from build123d import *

# Parameters (mm, degrees)
SKETCH1_W           = 15
SKETCH1_H           = 5
BOSS_EXTRUDE1_DEPTH = 9.75
SKETCH2_R           = 1.5
CUT_EXTRUDE1_DEPTH  = 4
SKETCH3_W           = 5
SKETCH3_H           = 0.5
BOSS_EXTRUDE2_DEPTH = 4
SKETCH4_W           = 5
SKETCH4_H           = 0.5
BOSS_EXTRUDE3_DEPTH = 4
SKETCH5_R           = 1
CUT_EXTRUDE2_DEPTH  = 4


with BuildPart() as part:
    # Sketch1 → Boss-Extrude1 (new body)
    with BuildSketch(Plane(origin=(0, 0, 0), x_dir=(1, 0, 0), z_dir=(0, 1, 0))):
        with Locations((-0.341726619, 0)):
            Rectangle(SKETCH1_W, SKETCH1_H)
    extrude(amount=BOSS_EXTRUDE1_DEPTH)

    # Sketch2 → Cut-Extrude1 (cut)
    with BuildSketch(Plane(origin=(0, 9.75, 0), x_dir=(1, 0, 0), z_dir=(0, 1, 0))):
        with Locations((-4.091726619, 0)):
            Circle(SKETCH2_R)
        with Locations((3.408273381, 0)):
            Circle(SKETCH2_R)
    extrude(amount=-CUT_EXTRUDE1_DEPTH, mode=Mode.SUBTRACT)

    # Sketch3 → Boss-Extrude2 (add)
    with BuildSketch(Plane(origin=(7.158273381, 0, 0), x_dir=(0, 0, -1), z_dir=(1, 0, 0))):
        with Locations((0, 0.25)):
            Rectangle(SKETCH3_W, SKETCH3_H)
    extrude(amount=BOSS_EXTRUDE2_DEPTH)

    # Sketch4 → Boss-Extrude3 (add)
    with BuildSketch(Plane.ZY.offset(7.841726619)):
        with Locations((0, 0.25)):
            Rectangle(SKETCH4_W, SKETCH4_H)
    extrude(amount=BOSS_EXTRUDE3_DEPTH)

    # Sketch5 → Cut-Extrude2 (cut)
    with BuildSketch(Plane(origin=(0, 0.5, 0), x_dir=(1, 0, 0), z_dir=(0, 1, 0))):
        with Locations((-9.841726619, 0)):
            Circle(SKETCH5_R)
        with Locations((9.158273381, 0)):
            Circle(SKETCH5_R)
    extrude(amount=-CUT_EXTRUDE2_DEPTH, mode=Mode.SUBTRACT)


solid = part.part
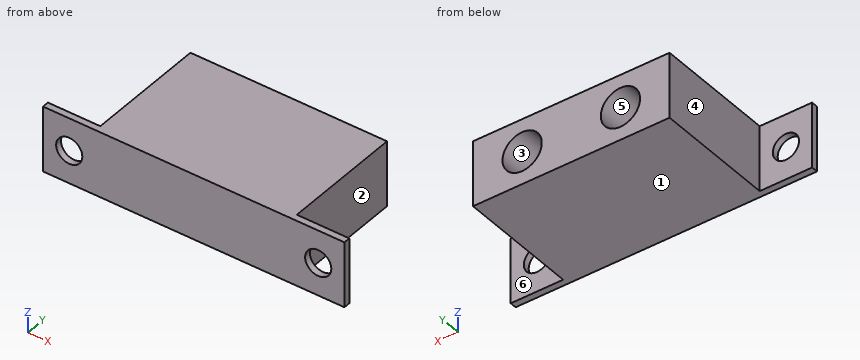
Geometry: final body of the model. Coordinates: model frame, mm. Face numbers are marked on the shaded views. A direction names the side the tool comes from. Give positions to 0.01 mm unless a question says otherwise; leave off trailing zeros. Write each loop counter-clockwise with the first axis right and the second up, starting at its lowest first coordinate (ties: lowest second). Pieces come first, ordered by that corner, then holes. Notation, with made-up numbers: M 22,23 L 51,23 A14 ccw 51,30 Z; hole C 88,32 d9. An arc over 180 degrees is marked long. Answer in a Markdown table with one row per item. Add a question column.
(1) Reachability of the marked faces 4, 5 and 6 from +Z, -Z, +X, -X, +Y, -Y: full face, straight path, thin tool, end or side. Return the list, or none.
(2) First-contact query: pin 1 (2.5 mm diameter, centred on x = 9.16, z = 0, fed in from +Y); pin 2 (2.5 mm diameter, centred on y = 6, z = -0.5, fed in from +X); pin 3 (2.5 mm diameter, centred on y = 3.5, z = -1, fed in from -X). Flat tips, straight axial feed; report the tip coordinate or a pass-through.
(3) Section B-B on y = 6.5. Return loops of the section in (x, z), and give its area (3 significant figures).
(4) Section C-C on z = -1.8. Return loops of the section in (x, y), and give its area (3 significant figures).
(5) Section D-D on y = 4. Return loops of the section in (x, z), and give its area (3 significant figures).
(6) Mould query, pull axis X, two halves, no side actions, for the marked faces 1, 2 and 3. Classes: +X half, -X half, draft (parallel to the pull), parting line (faces both ways), or undercut.
(7) Ray query, line 1 (X direction, y = 7, z = 0); line 2 (X direction, y = 0.45, z = 0); line 3 (Y direction, x = -10.5, z = -1.2). Return the intervals inside material, ascending.
(8) Section A-A on z = 0. Return loops of the section in (x, y).
Result set:
| question | item | result |
|---|---|---|
| 1 | face 4 | +Z, -Z, -X, +Y |
| 1 | face 5 | +Y |
| 1 | face 6 | +Z, -Z, +X, +Y |
| 2 | pin 1 | stops at y = 0.5 |
| 2 | pin 2 | stops at x = 7.16 |
| 2 | pin 3 | stops at x = -7.84 |
| 3 | outline | M -7.84,-2.5 L 7.16,-2.5 L 7.16,2.5 L -7.84,2.5 Z; hole C -4.09,0 d3; hole C 3.41,0 d3 |
| 3 | area | 60.9 mm^2 |
| 4 | outline | M -11.84,0 L 11.16,0 L 11.16,0.5 L 7.16,0.5 L 7.16,9.75 L -7.84,9.75 L -7.84,0.5 L -11.84,0.5 Z |
| 4 | area | 150 mm^2 |
| 5 | outline | M -7.84,-2.5 L 7.16,-2.5 L 7.16,2.5 L -7.84,2.5 Z |
| 5 | area | 75.0 mm^2 |
| 6 | face 1 | draft |
| 6 | face 2 | +X half |
| 6 | face 3 | undercut |
| 7 | line 1 | x = -7.84 to -5.59, -2.59 to 1.91, 4.91 to 7.16 |
| 7 | line 2 | x = -11.84 to -10.84, -8.84 to 8.16, 10.16 to 11.16 |
| 7 | line 3 | y = 0 to 0.5 |
| 8 | outline | M -11.84,0 L -10.84,0 L -10.84,0.5 L -11.84,0.5 Z; M -8.84,0 L 8.16,0 L 8.16,0.5 L 7.16,0.5 L 7.16,9.75 L 4.91,9.75 L 4.91,5.75 L 1.91,5.75 L 1.91,9.75 L -2.59,9.75 L -2.59,5.75 L -5.59,5.75 L -5.59,9.75 L -7.84,9.75 L -7.84,0.5 L -8.84,0.5 Z; M 10.16,0 L 11.16,0 L 11.16,0.5 L 10.16,0.5 Z |
